Geometry check sheet. Reference: the model listing, model coordinates, mm. Face numbers are marked on the shaded views. Round coordinates to 2 decimals unless told otherwise and drop trailing zeros. Write each loop counter-clockwise with the first axis right and the second up, starting at its lowest first coordinate (ties: lowest second). Pieces come first, ordered by that corner, then holes. Notation, with made-up numbers: (16.25, 7) -> (47.25, 7) arc R14 cw to (47.25, 23) -> close; hole circle Ø5 at (-21.75, 12). An arc over 180 degrees is marked (long way). One line per question, with ' | ' between items.
```python
from build123d import *

# Parameters (mm, degrees)
F1_DEPTH = 450.85


with BuildPart() as f1:
    # F0 (on Right) → F1 (new body)
    with BuildSketch(Plane.YZ):
        Polygon((133.195122, 31.0342), (63.725202, 15.262039), (67.190232, 0), (133.195122, 0), align=None)
        Polygon((38.1, 12.7), (0, 0), (10.040232, 0), (38.95556, 9.638443), (63.725202, 15.262039), (133.195122, 31.0342), (133.195122, 34.29), align=None)
    extrude(amount=-F1_DEPTH)


solid = f1.part
```
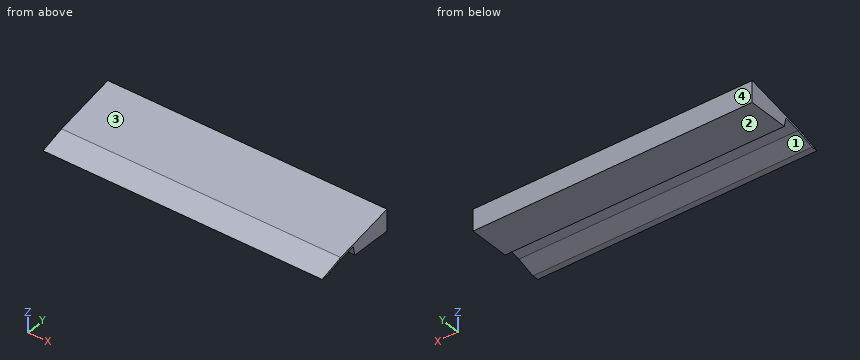
(1) Draft check along Y on the marked faces 1, 2, 3 and 4. Enter one of: +Y half, -Y half, draft (parallel to the pull), parting line (faces both ways), or undercut.
Resolved:
face 1: undercut | face 2: draft | face 3: -Y half | face 4: +Y half
(2) Material ranges on line 1 (Z direction, x = -429.5, y = 19); line 2 (Z direction, x = -212, y = 62), recorded low to high.
Resolved:
line 1: z = 2.99 to 6.33 | line 2: z = 14.87 to 18.13
(3) Sectioned sample at A-A on x = -380.5. Record the cut outline in (y, z), then the cut area to 3 significant figures.
Resolved:
outline: (0, 0) -> (10.04, 0) -> (38.96, 9.64) -> (63.73, 15.26) -> (67.19, 0) -> (133.2, 0) -> (133.2, 34.29) -> (38.1, 12.7) -> close | area: 2,000 mm2
(4) Sectioned sample at B-B on y = 29. Record the cut outline in (x, z).
Resolved:
outline: (-450.85, 6.32) -> (0, 6.32) -> (0, 9.67) -> (-450.85, 9.67) -> close
(5) Go/stop test with flat-tipped pins: pin 1 (1.5 mm diameter, centred on x = -157, y = 21, fed in from +Z); pin 2 (10 mm diameter, centred on x = -131, y = 43.5, fed in from +Z); pin 3 (3 mm diameter, centred on x = -332, y = 33, fed in from +Z). Record where each tip stops, or that it passes through.
Resolved:
pin 1: stops at z = 7.25 | pin 2: stops at z = 15.06 | pin 3: stops at z = 11.5
(6) Sectioned sample at C-C on z = 20. Record the cut outline in (x, y).
Resolved:
outline: (-450.85, 70.25) -> (0, 70.25) -> (0, 133.2) -> (-450.85, 133.2) -> close
